Can you work these out from the model? Positions are in its coordinate system, mm. Face numbers are marked on the shaded views. A direction names the side the tool comes from. Coordinates: 2 decimals unless noted, no trailing zeros. Order: outer loops, then holes, each group sorted by start corner. A loop starts at its lowest first (then second) coordinate and runs counter-clockwise, first axis right, second up. Notation, with made-up numbers: M 2,-32.5 L 10,-32.5 A22 ccw 10,-16.5 Z; hole C -4.5,22.25 d8. An arc over 180 degrees is marked long. Answer as CSV lines item,"result". Start each with the question number.
1. Will these pins go through, and if not, where does the flat tip stop? pin 1 (3 mm diameter, centred on x = 3, y = 13.5, fed in from -Z); pin 2 (2 mm diameter, centred on y = 12, z = -3, fed in from -X).
2. If we section it at C-C (y = 13.25): List the corners of the cut face in (x, z) for me.
3. If we section it at B-B (x = 2.9): List the corners of the cut face in (y, z) for me.
4. On a 3-axis mill with a long thin cutter (end or side, diameter ignored), from which of +Z, -Z, +X, -X, +Y, -Y can I reach the whole of each face in a straight line? I mean the marked faces 1, 2 and 3. Say none if no direction works.
5. If we section it at A-A (y = 4.75): List the corners of the cut face in (x, z) for me, plus the area to 3 significant figures.
6. I need wall thicknesses on line 1 along X through (y, z) = (4.05, -2.9); line 2 along Y through (x, z) = (3.25, 0); line 3 along Z through (x, y) = (2.35, 15.75). Which ranges of each line are inside material? Lowest first, please. Write a range as from..to.
7. If we section it at D-D (z = 2.75): List the corners of the cut face in (x, y) for me, plus the area to 3 significant figures.
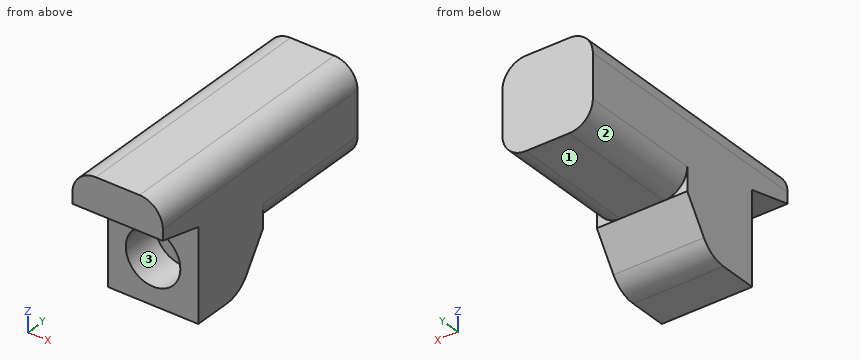
```python
from build123d import *

# Parameters (mm, degrees)
SKETCH_2_W               = 5.8
SKETCH_2_H               = 8.8
EXTRUDE_1_DEPTH          = 16.5
SKETCH_3_W               = 5.8
SKETCH_3_H               = 5.9
CUT_EXTRUDE_1_DEPTH      = 3
SKETCH_4_R               = 1.75
CUT_EXTRUDE_2_DEPTH      = 2.5
SKETCH_5_W               = 5.8
SKETCH_5_H               = 3
CUT_EXTRUDE_3_DEPTH      = 8
FILLET_1_R               = 1.5
CUT_EXTRUDE_4_DEPTH      = 19.426339843
CUT_EXTRUDE_4_DEPTH_BACK = 19.426339843
FILLET_2_R               = 2
CUT_EXTRUDE_5_DEPTH      = 19.426339843
CUT_EXTRUDE_5_DEPTH_BACK = 19.426339843


with BuildPart() as part:
    # ｽｹｯﾁ2 → ﾎﾞｽ - 押し出し1 (new body)
    with BuildSketch(Plane(origin=(0, 0, 0), x_dir=(1, 0, 0), z_dir=(0, 1, 0))):
        with Locations((2.9, 1.4)):
            Rectangle(SKETCH_2_W, SKETCH_2_H)
    extrude(amount=EXTRUDE_1_DEPTH)

    # ｽｹｯﾁ3 → ｶｯﾄ - 押し出し1 (cut)
    with BuildSketch(Plane.XZ):
        with Locations((2.9, -2.85)):
            Rectangle(SKETCH_3_W, SKETCH_3_H)
    extrude(amount=-CUT_EXTRUDE_1_DEPTH, mode=Mode.SUBTRACT)

    # ｽｹｯﾁ4 → ｶｯﾄ - 押し出し2 (cut)
    with BuildSketch(Plane.XZ.offset(-3)):
        with Locations(Location((2.9, -2.9, 0), (0, 0, 270))):
            Circle(SKETCH_4_R)
    extrude(amount=-CUT_EXTRUDE_2_DEPTH, mode=Mode.SUBTRACT)

    # ｽｹｯﾁ5 → ｶｯﾄ - 押し出し3 (cut)
    with BuildSketch(Plane(origin=(0, 16.5, 0), x_dir=(1, 0, 0), z_dir=(0, 1, 0))):
        with Locations((2.9, 4.3)):
            Rectangle(SKETCH_5_W, SKETCH_5_H)
    extrude(amount=-CUT_EXTRUDE_3_DEPTH, mode=Mode.SUBTRACT)

    # ﾌｨﾚｯﾄ1
    fillet_1_edges = [part.edges().sort_by_distance(p)[0] for p in [
        (0, 12.5, -2.8),
        (5.8, 12.5, -2.8),
        (5.8, 8.25, 3),
        (0, 8.25, 3),
    ]]
    fillet(fillet_1_edges, radius=FILLET_1_R)

    # ｽｹｯﾁ9 → ｶｯﾄ - 押し出し4 (cut, two sides: drawn at the far end of the back side and taken through both)
    with BuildSketch(Plane(origin=(5.8, 0, 0), x_dir=(0, 0, -1), z_dir=(1, 0, 0)).offset(-CUT_EXTRUDE_4_DEPTH_BACK)):
        Polygon((5.8, 8.5), (2.8, 8.5), (5.8, 6.5), align=None)
    extrude(amount=CUT_EXTRUDE_4_DEPTH + CUT_EXTRUDE_4_DEPTH_BACK, mode=Mode.SUBTRACT)

    # ﾌｨﾚｯﾄ2
    fillet_2_edges = [part.edges().sort_by_distance(p)[0] for p in [
        (2.9, 6.5, -5.8),
    ]]
    fillet(fillet_2_edges, radius=FILLET_2_R)

    # ｽｹｯﾁ10 → ｶｯﾄ - 押し出し5 (cut, two sides: drawn at the far end of the back side and taken through both)
    with BuildSketch(Plane(origin=(5.8, 0, 0), x_dir=(0, 0, -1), z_dir=(1, 0, 0)).offset(-CUT_EXTRUDE_5_DEPTH_BACK)):
        Polygon((-0.1, 0), (-0.1, 3), (-0.8, 0), align=None)
    extrude(amount=CUT_EXTRUDE_5_DEPTH + CUT_EXTRUDE_5_DEPTH_BACK, mode=Mode.SUBTRACT)


solid = part.part
```
Solved:
1,pin 1,"z = -2.8"
1,pin 2,"x = 0.17"
2,outline,"M 0,-1.3 A1.5 ccw 1.5,-2.8 L 4.3,-2.8 A1.5 ccw 5.8,-1.3 L 5.8,1.5 A1.5 ccw 4.3,3 L 1.5,3 A1.5 ccw 0,1.5 Z"
3,outline,"M 0,0.8 L 3,0.1 L 3,-1.15 L 5.5,-1.15 L 5.5,-4.65 L 3,-4.65 L 3,-5.8 L 5.43,-5.8 A2 ccw 7.09,-4.91 L 8.5,-2.8 L 16.5,-2.8 L 16.5,3 L 0,3 Z"
4,face 1,"-Z, +X, -X, +Y"
4,face 2,"-Z, -X, +Y"
4,face 3,"-Y"
5,outline,"M 0,-5.8 L 5.8,-5.8 L 5.8,1.5 A1.5 ccw 4.3,3 L 1.5,3 A1.5 ccw 0,1.5 Z; hole C 2.9,-2.9 d3.5"
5,area,"40.5 mm²"
6,line 1,"0..1.15, 4.65..5.8"
6,line 2,"3..16.5"
6,line 3,"-2.8..3"
7,outline,"M 0.67,0 L 5.13,0 L 5.13,16.5 L 0.67,16.5 Z"
7,area,"73.6 mm²"
